Could you check a few things on this drawing? It's one solid part, dimensions in mm from its lowest x, y, z. A direction names the side the tool comes from. Round coordinates to 2 decimals unless told otherwise and drop trailing zeros. Write each loop counter-clockwise with the first axis right and the second up, starting at its lowest first coordinate (ties: lowest second). Pieces come first, ordered by that corner, then holes. Notation, with made-up numbers: (31.25, 16.5) -> (52.25, 16.5) arc R27 cw to (52.25, 41.5) -> close; hole circle Ø1 at (13.5, -15.75). An arc over 180 degrees is marked (long way). Answer in a Markdown table with one row per item.
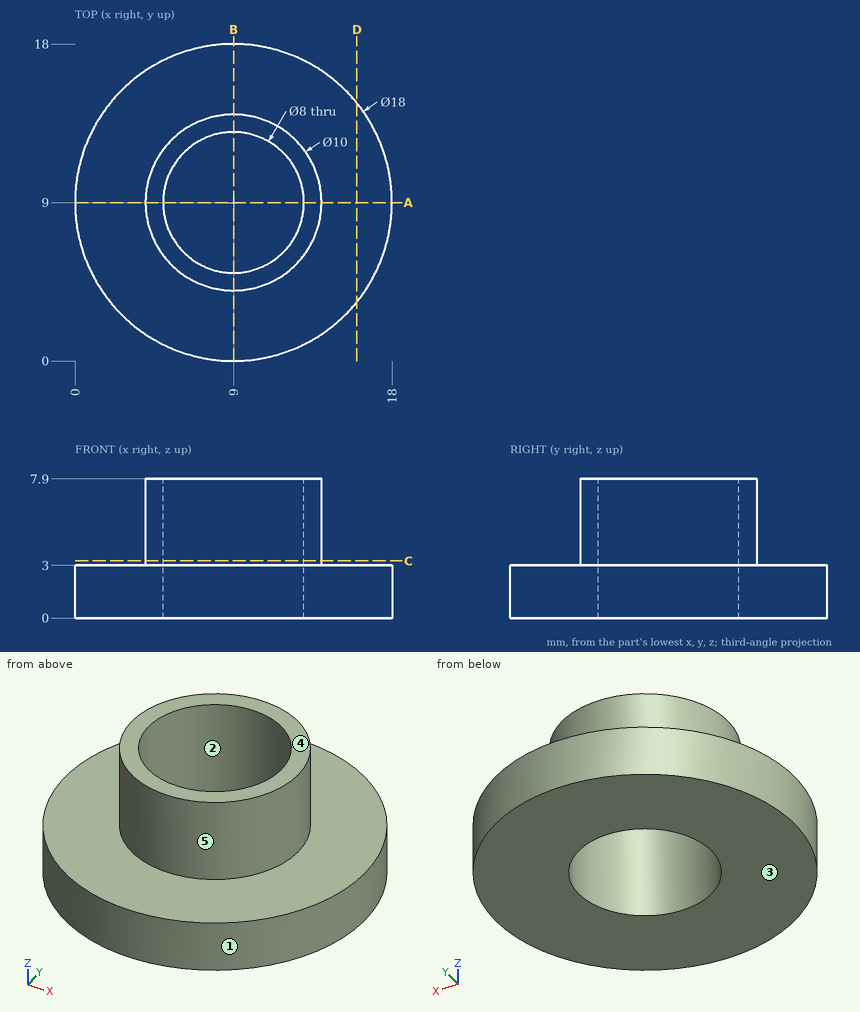
1) We'd pull the mould along Y, two halves only. Please class the marked faces 1, 2 and 3: +Y half, -Y half, draft (parallel to the pull), parting line (faces both ways), or undercut.
Response:
| item | result |
|---|---|
| face 1 | parting line |
| face 2 | undercut |
| face 3 | draft |
2) I want a section at A-A, the plane y = 9. List the corners of the cut face in (x, z) for me.
Response:
| item | result |
|---|---|
| outline | (0, 0) -> (5, 0) -> (5, 7.9) -> (4, 7.9) -> (4, 3) -> (0, 3) -> close; (13, 0) -> (18, 0) -> (18, 3) -> (14, 3) -> (14, 7.9) -> (13, 7.9) -> close |
3) I want a section at D-D, the plane x = 16. List the corners of the cut face in (y, z) for me.
Response:
| item | result |
|---|---|
| outline | (3.34, 0) -> (14.66, 0) -> (14.66, 3) -> (3.34, 3) -> close |
4) For pin 1 (2 mm diameter, centred on x = 5.5, z = 4.5, fed in from +Y); pin 2 (4 mm diameter, centred on x = 7.5, z = 6, fed in from -Y); pin 3 (1.5 mm diameter, centred on y = 8, z = 3.5, fed in from -X), each with a flat end and sliding along its axis, tell me the tip position at first contact or that it passes through.
Response:
| item | result |
|---|---|
| pin 1 | stops at y = 13.33 |
| pin 2 | stops at y = 4 |
| pin 3 | stops at x = 0.01 |
5) Which directions (+Z, -Z, +X, -X, +Y, -Y) give clear straight access to the entire face, cutting with the end or side of a thin tool? Please do the marked faces 4 and 5.
Response:
| item | result |
|---|---|
| face 4 | +Z, +X, -X, +Y, -Y |
| face 5 | +Z |
6) I want a section at C-C, the plane z = 3.25. List the corners of the cut face in (x, y) for me.
Response:
| item | result |
|---|---|
| outline | circle Ø10 at (9, 9); hole circle Ø8 at (9, 9) |
7) I need wall thicknesses on line 1 (Y direction, x = 9, z = 4); line 2 (Z direction, x = 16.75, y = 7.75); line 3 (X direction, y = 10.5, z = 3.5). Which ranges of each line are inside material? Lowest first, please. Write a range as [from, to].
Response:
| item | result |
|---|---|
| line 1 | y = [4, 5], [13, 14] |
| line 2 | z = [0, 3] |
| line 3 | x = [4.23, 5.29], [12.71, 13.77] |
